Answer from the drawing. Dimensions are ordinates in mm from the lowest x, y and z of the part. A direction names the side the tool comes from. Give positions to 0.01 mm unless a question says otherwise; leave off trailing zeros. Loops run counter-clockwise (first coordinate to the right, second up) from the corner with the lowest first, then second, coordinate; pieces in that order, holes last. Notation, with made-up numbers: (1, 89) - (42, 89) arc R17 cw to (42, 96) - close; hole circle Ø5 at (4.25, -30). An arc over 180 degrees is marked (long way). Answer as CSV lines item,"result". Start each with the question number.
1) A cutting plane is placed at A-A (x = 6). Determine the outline of the cut face in (y, z), and give its area (3 significant figures).
2) A cutting plane is placed at D-D (y = 2). Determine the outline of the cut face in (x, z).
3) Flat-ended cylindrical pins translate along their axes: pin 1 (5 mm diameter, centred on x = 8, y = 2.5, fed in from -Z); pin 2 (0.5 mm diameter, centred on x = 6, y = 1, fed in from +Z); pin 3 (0.5 mm diameter, centred on y = 11, z = 4.5, fed in from -X); pin 4 (0.8 mm diameter, centred on y = 2, z = 4.5, fed in from +X). Find the tip coordinate at first contact, or state that the pin passes through.
4) A cutting plane is placed at C-C (z = 3.2). Determine the outline of the cut face in (x, y).
5) Find the intervals of material crossed by line 1 along Y through (x, z) = (6, 2); line 2 along X through (y, z) = (5.25, 1.8), in increasing order.
6) For a pull along Y with two mould halves and no side action, classify the marked faces 3, 4 and 5 as pulls with the +Y half, pulls with the -Y half, needs draft (parallel to the pull), parting line crosses it, or undercut.
7) For the marked faces 1 and 2, determine the directions among +Z, -Z, +X, -X, +Y, -Y from which every point of the face is accessible in a straight line to the end or side of a thin tool.
8) A cutting plane is placed at B-B (y = 6). Determine the outline of the cut face in (x, z).
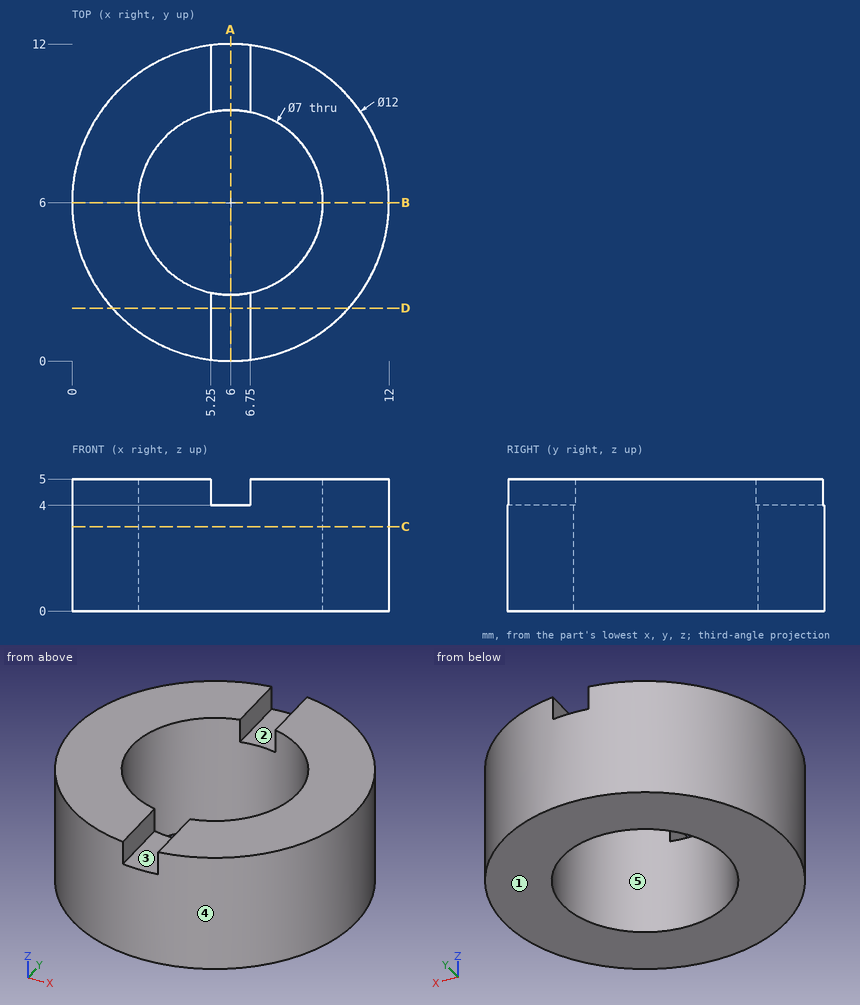
Ans:
1,outline,"(0, 0) - (2.5, 0) - (2.5, 4) - (0, 4) - close; (9.5, 0) - (12, 0) - (12, 4) - (9.5, 4) - close"
1,area,"20.0 mm2"
2,outline,"(1.53, 0) - (10.47, 0) - (10.47, 5) - (6.75, 5) - (6.75, 4) - (5.25, 4) - (5.25, 5) - (1.53, 5) - close"
3,pin 1,"z = 0"
3,pin 2,"z = 4"
3,pin 3,"x = 2.33"
3,pin 4,"x = 10.8"
4,outline,"circle Ø12 at (6, 6); hole circle Ø7 at (6, 6)"
5,line 1,"0 to 2.5, 9.5 to 12"
5,line 2,"0.05 to 2.58, 9.42 to 11.95"
6,face 3,"needs draft"
6,face 4,"parting line crosses it"
6,face 5,"undercut"
7,face 1,"-Z, +X, -X, +Y, -Y"
7,face 2,"+Z, +Y, -Y"
8,outline,"(0, 0) - (2.5, 0) - (2.5, 5) - (0, 5) - close; (9.5, 0) - (12, 0) - (12, 5) - (9.5, 5) - close"
